```python
from build123d import *
from build123d.topology import SkipClean

# Parameters (mm, degrees)
SKETCH1_W           = 60
SKETCH1_H           = 25
BOSS_EXTRUDE1_DEPTH = 4
SKETCH2_W           = 40
SKETCH2_H           = 1
BOSS_EXTRUDE2_DEPTH = 2.5146
SKETCH3_W           = 40
SKETCH3_H           = 1
BOSS_EXTRUDE3_DEPTH = 1


with BuildPart() as part:
    # Sketch1 → Boss-Extrude1 (new body)
    with BuildSketch(Plane.XY):
        with Locations((4.416243655, 2.220812183)):
            Rectangle(SKETCH1_W, SKETCH1_H)
    extrude(amount=BOSS_EXTRUDE1_DEPTH)

    # Sketch2 → Boss-Extrude2 (add)
    with BuildSketch(Plane(origin=(0, 0, 0), x_dir=(-1, 0, 0), z_dir=(0, 0, -1))):
        with Locations((-14.416243533, -7.279192817)):
            Rectangle(SKETCH2_W, SKETCH2_H)
    extrude(amount=BOSS_EXTRUDE2_DEPTH)

    # Sketch3 → Boss-Extrude3 (add)
    with SkipClean():  # the faces are left unmerged after this step: merging them gives an invalid solid
        with BuildSketch(Plane(origin=(0, 0, 0), x_dir=(-1, 0, 0), z_dir=(0, 0, -1))):
            with Locations((-14.416243533, -4.279192817)):
                Rectangle(SKETCH3_W, SKETCH3_H)
        extrude(amount=BOSS_EXTRUDE3_DEPTH)


solid = part.part
```
Could you check a few things on this model? Use its own coordinates, in mm. A direction names the side the tool comes from. Round coordinates to 2 decimals unless told otherwise and drop trailing zeros. Loops run counter-clockwise (first coordinate to the right, second up) from the corner with the lowest first, then second, coordinate; pieces in that order, holes last. Notation, with made-up numbers: (31.5, 62.5) - (73.5, 62.5) arc R16 ccw to (73.5, 78.5) - close; hole circle Ø2 at (74.5, 54.5). An arc over 180 degrees is marked (long way). Use CSV: the item, a comma, the result in double quotes.
Item 1: I need wall thicknesses on L1, parallel to Z at x = 21, y = 6; L2, parallel to Z at x = 13, y = -4.5. Which ranges of each line are inside material? Lowest first, please. Write a range as [from, to].
Here are the results:
L1,"z = [0, 4]"
L2,"z = [-1, 4]"
Item 2: If we section it at A-A on x = 27.5: List the corners of the cut face in (y, z) for me.
Here are the results:
outline,"(-10.28, 0) - (-7.78, 0) - (-7.78, -2.51) - (-6.78, -2.51) - (-6.78, 0) - (-4.78, 0) - (-4.78, -1) - (-3.78, -1) - (-3.78, 0) - (14.72, 0) - (14.72, 4) - (-10.28, 4) - close"
Item 3: If we section it at B-B on y = 8: List the corners of the cut face in (x, z) for me.
Here are the results:
outline,"(-25.58, 0) - (34.42, 0) - (34.42, 4) - (-25.58, 4) - close"
Item 4: For faces 4 (the flat face through (14.7, -4.779, -0.5)), 5 (the flat face through (15, -7.779, -1)), 6 (the flat face through (-5.584, -4.3, -0.5)), which set-ups out of +Z, -Z, +X, -X, +Y, -Y let a thin tool reach every point of the face, with its end or its side?
Here are the results:
face 4,"-Z, +X, -X"
face 5,"-Z, +X, -X, -Y"
face 6,"-Z, -X, +Y, -Y"
Item 5: If we mould it in two halves opening along Y, with no side actions, what happens to faces 1 (the flat face through (15, -4, -1)), 2 (the flat face through (4, 14.721, 2)), 3 (the flat face through (15, -6.779, -1))? For each: pulls with the +Y half, pulls with the -Y half, needs draft (parallel to the pull), parting line crosses it, or undercut.
Here are the results:
face 1,"needs draft"
face 2,"pulls with the +Y half"
face 3,"undercut"
Item 6: Will these pins go through, and if not, where does the flat tip stop? pin 1 (0.8 mm diameter, centred on x = 21, z = -1.5, fed in from +Y); pin 2 (1.5 mm diameter, centred on x = -9.5, y = -4, fed in from -Z); pin 3 (0.8 mm diameter, centred on x = 24.5, z = -0.5, fed in from +Y).
Here are the results:
pin 1,"stops at y = -6.78"
pin 2,"stops at z = 0"
pin 3,"stops at y = -3.78"
